Autodesk Inventor part; units mm, degrees
ref_plane "YZ Plane" through (0, 0, 0) normal (1, 0, 0) x (0, 1, 0)
ref_plane "XZ Plane" through (0, 0, 0) normal (0, 1, 0) x (-1, 0, 0)
ref_plane "XY Plane" through (0, 0, 0) normal (0, 0, 1) x (1, 0, 0)
sketch "Эскиз1" plane through (0, 0, 0) normal (0, 1, 0) x (-1, 0, 0)
  line L0 (26, 25) -> (-26, 25)
  line L1 (-26, 25) -> (-26, -25)
  line L2 (-26, -25) -> (26, -25)
  line L3 (26, -25) -> (26, 25)
  line L4 (36.4, 0) -> (-36.4, 0)
  line L5 (0, -35) -> (0, 35)
  point P0 (0, 0)
  dimension "d0" = 52
  dimension "d1" = 50
extrude "Выдавливание1" add sketch "Эскиз1" along normal blind 11
shell "Оболочка1" thickness 1 removed faces 1 at (-8.6667, 11, -8.3333)
sketch "Эскиз2" plane through (-26, 0, -25) normal (-1, 0, 0) x (0, 0, 1)
  line L0 (28.9, 7.4) -> (21.1, 7.4)
  line L1 (21.1, 7.4) -> (21.1, 11)
  line L2 (21.1, 11) -> (28.9, 11)
  line L3 (28.9, 11) -> (28.9, 7.4)
  line L4 (0, 0) -> (50, 0)
  line L5 (25, -2.2) -> (25, 13.2)
  line L6 (0, 11) -> (50, 11)
  point P0 (25, 0)
  dimension "d5" = 7.4
  dimension "d7" = 7.8
extrude "Выдавливание2" cut sketch "Эскиз2" against normal up to surface (1 mm away)
fillet "Сопряжение1" radius 1.5 2 edges at (-25.5, 7.4, -3.9) (-25.5, 7.4, 3.9)
fillet "Сопряжение2" radius 2 4 edges at (25, 6, 24) (25, 6, -24) (-25, 6, -24) (-25, 6, 24)
sketch "Эскиз4" plane through (25, 1, -22) normal (-1, 0, 0) x (0, 0, 1)
  line L0 (44, 0) -> (0, 0)
  line L1 (24, 0) -> (20, 0)
  line L2 (20, 0) -> (20, 4)
  line L3 (20, 4) -> (24, 4)
  line L4 (24, 4) -> (24, 0)
  line L5 (22, -3.2) -> (22, 12.2)
  point P0 (22, -1)
  dimension "d16" = 4
  dimension "d17" = 4
extrude "Выдавливание4" cut sketch "Эскиз4" against normal through all
sketch "Эскиз5" plane through (-23, 1, 24) normal (0, 1, 0) x (1, 0, 0)
  line L0 (48, 26) -> (48, 22) construction
  circle A0 centre (48, 24) radius 7 construction
  line L1 (48, 26) -> (48, 46) construction
  line L2 (48, 26.75) -> (41, 26.75) construction
  line L3 (41, 26.75) -> (41, 21.25) construction
  line L4 (41, 21.25) -> (48, 21.25) construction
  line L5 (48, 21.25) -> (48, 26.75) construction
  line L6 (-14.64, 24) -> (66.84, 24) construction
  line L7 (48, 2) -> (48, 22) construction
  line L8 (41, 21.25) -> (48, 21.25) construction
  line L9 (48, 21.25) -> (48, 20.25) construction
  line L10 (48, 20.25) -> (41, 20.25) construction
  line L11 (41, 20.25) -> (41, 21.25) construction
  line L12 (41, 26.75) -> (48, 26.75) construction
  line L13 (48, 26.75) -> (48, 27.75) construction
  line L14 (48, 27.75) -> (41, 27.75) construction
  line L15 (41, 27.75) -> (41, 26.75) construction
  arc A1 (42.1104, 21.25) -> (42.6908, 20.25) centre (48, 24) ccw
  arc A2 (42.6908, 27.75) -> (42.1104, 26.75) centre (48, 24) ccw
  arc A3 (42.1104, 26.75) -> (42.1104, 21.25) centre (48, 24) ccw
  arc A4 (43.2369, 26.75) -> (43.2369, 21.25) centre (48, 24) ccw
  line L16 (43.2369, 26.75) -> (48, 26.75)
  line L17 (48, 26.75) -> (48, 27.75)
  line L18 (48, 27.75) -> (42.6908, 27.75)
  line L19 (43.2369, 21.25) -> (48, 21.25)
  line L20 (48, 21.25) -> (48, 20.25)
  line L21 (42.6908, 20.25) -> (48, 20.25)
  point P0 (23, 24)
  dimension "d20" = 14
  dimension "d21" = 5.5
  dimension "d22" = 1
  dimension "d23" = 1
  dimension "d24" = 0.5
  dimension "d25" = 1
extrude "Выдавливание5" add sketch "Эскиз5" along normal blind 5
sketch "Эскиз8" plane through (-23, 1, -24) normal (0, 1, 0) x (1, 0, 0)
  line L0 (1.875, -4.025) -> (44.125, -4.025) construction
  line L1 (44.125, -4.025) -> (44.125, -43.975) construction
  line L2 (44.125, -43.975) -> (1.875, -43.975) construction
  line L3 (1.875, -43.975) -> (1.875, -4.025) construction
  line L4 (23, 11) -> (23, -59) construction
  line L5 (-13.4, -24) -> (59.4, -24) construction
  circle A0 centre (1.875, -4.025) radius 1.35
  circle A1 centre (44.125, -4.025) radius 1.35
  circle A2 centre (1.875, -43.975) radius 1.35
  circle A3 centre (44.125, -43.975) radius 1.35
  point P0 (23, -24)
  dimension "d33" = 42.25
  dimension "d34" = 39.95
  dimension "d35" = 2.7
extrude "Выдавливание7" cut sketch "Эскиз8" against normal through all
properties part number "BOTTOM"
Geometry: final body of the model. Coordinates: model frame, mm. A direction names the side the tool comes from. Coordinates: 2 decimals unless noted, no trailing zeros. Loops run counter-clockwise (first coordinate to the right, second up) from the corner with the lowest first, then second, coordinate; pieces in that order, holes last. Notation, with made-up numbers: (-10, -13.75) -> (44, -13.75) arc R7 cw to (44, -4.75) -> close; hole circle Ø9 at (-5.75, 38.25). An arc over 180 degrees is marked (long way). Use a Markdown table: item, result. Add a question column.
(1) Section query C-C, the plane z = -13.5. Return loops of the section in (x, y), plus the area to 3 significant figures.
(2) Line query: line 1 along Z through (x, y) = (23, 1.5); line 2 along Z through (x, y) = (1, 3); line 3 along X through (y, z) = (1.25, -13.5). Output: solid intervals per line, ascending.
(3) Access query for faces 4 (the flat face through (0, 0, 0)), 5 (the cylindrical face through (-24.43, 5.93, -23.4)), 6 (the cylindrical face through (-25.49, 7.85, 3.47)). Directions: +Z, -Z, +X, -X, +Y, -Y. A direction counts if a zero-diameter tool reaches every point of the face in a straight line with its end or side. Return the directions, or none.
(4) Section query B-B, the plane x = 6.5. Return loops of the section in (y, z), plus the area to 3 significant figures.
(5) Section query D-D, the plane y = 9.5. Return loops of the section in (x, z).
(6) Pin query (flat end, axial travel): pin 1 Ø10 at (x, z) = (18, -10.5) entering from -Y; pin 2 Ø2 at (x, z) = (6, -12) entering from +Y; pin 3 Ø3 at (x, z) = (20.5, 0) entering from +Y; pin 4 Ø2 at (x, z) = (-21.125, -19.975) entering from +Y. Return the tip coordinate at first contact, or that it passes through.
(7) Section query A-A, the plane y = 3.25. Return loops of the section in (x, z).
(8) Mould query, pull axis X, two halves, no side actions, for faces 1 (the flat face through (23, 3, 2.75)), 2 (the flat face through (-26, 5, 0)), 3 (the cylindrical face through (-25.49, 7.83, -3.45)). Classes: pulls with the +X half, pulls with the -X half, needs draft (parallel to the pull), parting line crosses it, or undercut.
Answer:
| question | item | result |
|---|---|---|
| 1 | outline | (-26, 0) -> (26, 0) -> (26, 11) -> (25, 11) -> (25, 1) -> (-25, 1) -> (-25, 11) -> (-26, 11) -> close |
| 1 | area | 72.0 mm^2 |
| 2 | line 1 | z = -25 to -24, -3.75 to -2.75, 2.75 to 3.75, 24 to 25 |
| 2 | line 2 | z = -25 to -24, 24 to 25 |
| 2 | line 3 | x = -26 to -25, 25 to 26 |
| 3 | face 4 | +Z, -Z, +X, -X, -Y |
| 3 | face 5 | +Y |
| 3 | face 6 | -X, +Y |
| 4 | outline | (0, -25) -> (11, -25) -> (11, -24) -> (1, -24) -> (1, 24) -> (11, 24) -> (11, 25) -> (0, 25) -> close |
| 4 | area | 70.0 mm^2 |
| 5 | outline | (-26, -25) -> (26, -25) -> (26, 25) -> (-26, 25) -> (-26, 3.9) -> (-25, 3.9) -> (-25, 22) arc R2 cw to (-23, 24) -> (23, 24) arc R2 cw to (25, 22) -> (25, -22) arc R2 cw to (23, -24) -> (-23, -24) arc R2 cw to (-25, -22) -> (-25, -3.9) -> (-26, -3.9) -> close |
| 6 | pin 1 | stops at y = 0 |
| 6 | pin 2 | stops at y = 1 |
| 6 | pin 3 | stops at y = 6 |
| 6 | pin 4 | passes through |
| 7 | outline | (-26, -25) -> (26, -25) -> (26, -2) -> (25, -2) -> (25, -2.75) -> (20.24, -2.75) arc R5.5 cw to (20.24, 2.75) -> (25, 2.75) -> (25, 2) -> (26, 2) -> (26, 25) -> (-26, 25) -> close; hole (-25, -22) arc R2 ccw to (-23, -24) -> (23, -24) arc R2 ccw to (25, -22) -> (25, -3.75) -> (19.69, -3.75) arc R6.5 cw to (19.11, -2.75) arc R6.5 cw to (19.11, 2.75) arc R6.5 cw to (19.69, 3.75) -> (25, 3.75) -> (25, 22) arc R2 ccw to (23, 24) -> (-23, 24) arc R2 ccw to (-25, 22) -> close |
| 8 | face 1 | undercut |
| 8 | face 2 | pulls with the -X half |
| 8 | face 3 | needs draft |
